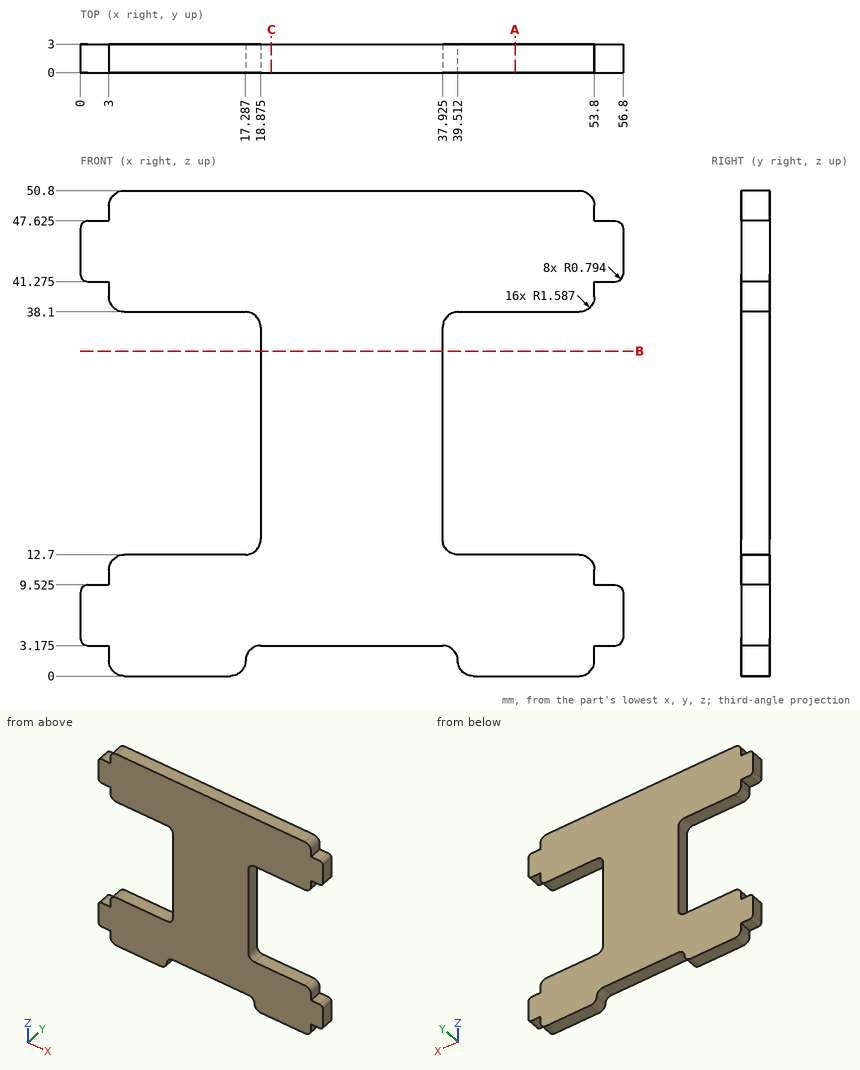
Input: dimensioned drawing with shaded views. Units: mm. Origin: part minimum x, y, z. Coordinates: 2 decimals unless noted, no trailing zeros. Write each loop counter-clockwise with the first axis right and the second up, starting at its lowest first coordinate (ties: lowest second). Pieces come first, ordered by that corner, then holes. Notation, with made-up numbers: M 54,4.25 L 88,4.25 A11 cw 88,25.25 Z; hole C 56.5,-14.5 d1. An arc over 180 degrees is marked long. Answer as a JSON object with one key per item and string values. Group by question number.
(1) Ray query, line 1 along Z through (x, y) = (10, 2.6); line 2 along Z through (x, y) = (54.5, 2.8) (1 decimal); line 3 along Z through (x, y) = (27.5, 0.2) (1 decimal). Return the intervals inside material, ascending. Write a range as [from, to].
(2) Section C-C on x = 20. Output: boundary loops of the cut face in (y, z) (1 decimal).
(3) Section B-B on z = 34. Output: boundary loops of the cut face in (x, y) (1 decimal).
(4) Section A-A on x = 45.5. Output: boundary loops of the cut face in (y, z).
(5) Contact query for flat-ended pins moving along their axis: P1, Ø0.5, axis at y = 1.5, z = 2.5, coming from the +X side; P2, Ø1.1, axis at x = 54.5, y = 1, coming from the -Z side (1 decimal); P3, Ø1.5, axis at y = 1, z = 27.5, coming from the +X side (1 decimal); P4, Ø1.5, axis at x = 13, z = 36.5, coming from the +Y side. Output: stop coordinate, or through.
Result set:
{
 "1": {"line 1": "z = [0, 12.7], [38.1, 50.8]", "line 2": "z = [3.2, 9.5], [41.3, 47.6]", "line 3": "z = [3.2, 50.8]"},
 "2": {"outline": "M 0,3.2 L 3,3.2 L 3,50.8 L 0,50.8 Z"},
 "3": {"outline": "M 18.9,0 L 37.9,0 L 37.9,3 L 18.9,3 Z"},
 "4": {"outline": "M 0,0 L 3,0 L 3,12.7 L 0,12.7 Z; M 0,38.1 L 3,38.1 L 3,50.8 L 0,50.8 Z"},
 "5": {"P1": "stops at x = 53.8", "P2": "stops at z = 3.2", "P3": "stops at x = 37.9", "P4": "passes through"}
}
